The listing builds one solid part. Answer for the finished solid, in the listing's coordinates (mm). Face numbers are marked on the shaded views. A direction names the side the tool comes from. Give positions to 0.01 mm unless a question says otherwise; leave off trailing zeros. Write each loop counter-clockwise with the first axis right and the second up, starting at its lowest first coordinate (ties: lowest second). Pieces come first, ordered by that corner, then holes. Notation, with made-up numbers: M 52,71.5 L 75,71.5 A23 ccw 75,99.5 Z; hole C -15,33 d10. An arc over 180 degrees is marked long. Return JSON: item names as keys, results as strings.
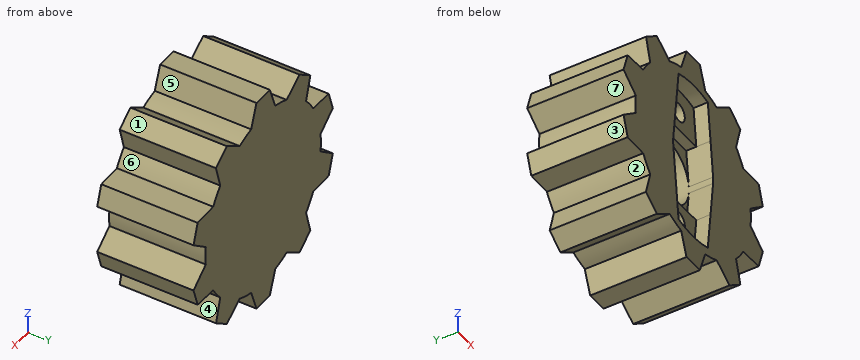
from build123d import *

# Parameters (mm, degrees)
CROQUIS1_R              = 3.75
SALIENTE_EXTRUIR1_DEPTH = 11.5
CROQUIS1_4_R            = 1.1
CORTAR_EXTRUIR1_DEPTH   = 1.7
CORTAR_EXTRUIR2_START   = 1.7
CORTAR_EXTRUIR2_DEPTH   = 1.2
CUT_EXTRUDE1_START      = 1.7
CROQUIS1_7_R            = 1.1
CUT_EXTRUDE1_DEPTH      = 6.5
BOSS_EXTRUDE1_START     = 11.5
BOSS_EXTRUDE1_DEPTH     = 5.6


with BuildPart() as part:
    # Croquis1 → Saliente-Extruir1 (new body)
    with BuildSketch(Plane(origin=(0, 0, 0), x_dir=(1, 0, 0), z_dir=(0, 1, 0))):
        with BuildLine():
            Line((1.248257156, 13.300370373), (-1.251742735, 13.299629349))
            Line((-1.251742735, 13.299629349), (-2.247599184, 10.563536241))
            ThreePointArc((-2.247599184, 10.563536241), (-3.339078028, 10.270859649), (-4.394000333, 9.865736722))
            Line((-4.394000333, 9.865736722), (-6.807900303, 11.493932811))
            Line((-6.807900303, 11.493932811), (-8.830007137, 10.023870243))
            Line((-8.830007137, 10.023870243), (-8.027436751, 7.224974686))
            ThreePointArc((-8.027436751, 7.224974686), (-8.7384307, 6.346639181), (-9.353755491, 5.398820076))
            Line((-9.353755491, 5.398820076), (-12.263671238, 5.297203579))
            Line((-12.263671238, 5.297203579), (-13.035508935, 2.919333403))
            Line((-13.035508935, 2.919333403), (-10.741066321, 1.126718369))
            ThreePointArc((-10.741066321, 1.126718369), (-10.799999853, -0.001781739), (-10.740693974, -1.13026234))
            Line((-10.740693974, -1.13026234), (-13.035136587, -2.922877375))
            Line((-13.035136587, -2.922877375), (-12.261889379, -5.300289572))
            Line((-12.261889379, -5.300289572), (-9.351973632, -5.401906069))
            ThreePointArc((-9.351973632, -5.401906069), (-8.73633614, -6.349522096), (-8.025052421, -7.227622959))
            Line((-8.025052421, -7.227622959), (-8.827622808, -10.026518516))
            Line((-8.827622808, -10.026518516), (-6.804644848, -11.495382082))
            Line((-6.804644848, -11.495382082), (-4.390744878, -9.867185993))
            ThreePointArc((-4.390744878, -9.867185993), (-3.335688959, -10.271960824), (-2.244113605, -10.564277265))
            Line((-2.244113605, -10.564277265), (-1.248257156, -13.300370373))
            Line((-1.248257156, -13.300370373), (1.251742735, -13.299629349))
            Line((1.251742735, -13.299629349), (2.247599184, -10.563536241))
            ThreePointArc((2.247599184, -10.563536241), (3.339078028, -10.270859649), (4.394000333, -9.865736722))
            Line((4.394000333, -9.865736722), (6.807900303, -11.493932811))
            Line((6.807900303, -11.493932811), (8.830007137, -10.023870243))
            Line((8.830007137, -10.023870243), (8.027436751, -7.224974686))
            ThreePointArc((8.027436751, -7.224974686), (8.7384307, -6.346639181), (9.353755491, -5.398820076))
            Line((9.353755491, -5.398820076), (12.263671238, -5.297203579))
            Line((12.263671238, -5.297203579), (13.035508935, -2.919333403))
            Line((13.035508935, -2.919333403), (10.741066321, -1.126718369))
            ThreePointArc((10.741066321, -1.126718369), (10.799999853, 0.001781739), (10.740693974, 1.13026234))
            Line((10.740693974, 1.13026234), (13.035136587, 2.922877375))
            Line((13.035136587, 2.922877375), (12.261889379, 5.300289572))
            Line((12.261889379, 5.300289572), (9.351973632, 5.401906069))
            ThreePointArc((9.351973632, 5.401906069), (8.73633614, 6.349522096), (8.025052421, 7.227622959))
            Line((8.025052421, 7.227622959), (8.827622808, 10.026518516))
            Line((8.827622808, 10.026518516), (6.804644848, 11.495382082))
            Line((6.804644848, 11.495382082), (4.390744878, 9.867185993))
            ThreePointArc((4.390744878, 9.867185993), (3.335688959, 10.271960824), (2.244113605, 10.564277265))
            Line((2.244113605, 10.564277265), (1.248257156, 13.300370373))
        make_face()
        with Locations(Location((0, 0, 0), (0, 0, 270))):
            Circle(CROQUIS1_R, mode=Mode.SUBTRACT)
    extrude(amount=SALIENTE_EXTRUIR1_DEPTH)

    # Croquis1<4> → Cortar-Extruir1 (cut)
    with BuildSketch(Plane(origin=(0, 0, 0), x_dir=(1, 0, 0), z_dir=(0, 1, 0))):
        with BuildLine():
            ThreePointArc((3.727502093, -0.41015625), (0, -3.75), (-3.727502093, -0.41015625))
            Line((-3.727502093, -0.41015625), (-3.249966737, -4.75))
            Line((-3.249966737, -4.75), (3.249966737, -4.75))
            Line((3.249966737, -4.75), (3.727502093, -0.41015625))
        make_face()
        with BuildLine():
            Line((3.249966737, -4.75), (-3.249966737, -4.75))
            Line((-3.249966737, -4.75), (-2.737205389, -9.409977746))
            ThreePointArc((-2.737205389, -9.409977746), (0, -9.7999987), (2.737205389, -9.409977746))
            Line((2.737205389, -9.409977746), (3.249966737, -4.75))
        make_face()
        with Locations((0, -7)):
            Circle(CROQUIS1_4_R, mode=Mode.SUBTRACT)
        with BuildLine():
            Line((3.248223947, 4.75), (-3.251709526, 4.75))
            Line((-3.251709526, 4.75), (-3.727664518, 0.408677426))
            ThreePointArc((-3.727664518, 0.408677426), (-0.001487905, 3.749999705), (3.727339039, 0.411635384))
            Line((3.727339039, 0.411635384), (3.248223947, 4.75))
        make_face()
        with BuildLine():
            Line((-2.740938342, 9.408891089), (-3.251709526, 4.75))
            Line((-3.251709526, 4.75), (3.248223947, 4.75))
            Line((3.248223947, 4.75), (2.733471058, 9.411063197))
            ThreePointArc((2.733471058, 9.411063197), (-0.003888392, 9.799997928), (-2.740938342, 9.408891089))
        make_face()
        with Locations((0, 7)):
            Circle(CROQUIS1_4_R, mode=Mode.SUBTRACT)
        with Locations((0, 7)):
            Circle(CROQUIS1_4_R)
        with Locations((0, -7)):
            Circle(CROQUIS1_4_R)
    extrude(amount=CORTAR_EXTRUIR1_DEPTH, mode=Mode.SUBTRACT)

    # Croquis1<5> → Cortar-Extruir2 (cut)
    with BuildSketch(Plane(origin=(0, 0, 0), x_dir=(1, 0, 0), z_dir=(0, 1, 0)).offset(CORTAR_EXTRUIR2_START)):
        with BuildLine():
            Line((3.248223947, 4.75), (-3.251709526, 4.75))
            Line((-3.251709526, 4.75), (-3.727664518, 0.408677426))
            ThreePointArc((-3.727664518, 0.408677426), (-0.001487905, 3.749999705), (3.727339039, 0.411635384))
            Line((3.727339039, 0.411635384), (3.248223947, 4.75))
        make_face()
        with BuildLine():
            ThreePointArc((3.727502093, -0.41015625), (0, -3.75), (-3.727502093, -0.41015625))
            Line((-3.727502093, -0.41015625), (-3.249966737, -4.75))
            Line((-3.249966737, -4.75), (3.249966737, -4.75))
            Line((3.249966737, -4.75), (3.727502093, -0.41015625))
        make_face()
    extrude(amount=CORTAR_EXTRUIR2_DEPTH, mode=Mode.SUBTRACT)

    # Croquis1<7> → Cut-Extrude1 (cut)
    with BuildSketch(Plane(origin=(0, 0, 0), x_dir=(1, 0, 0), z_dir=(0, 1, 0)).offset(CUT_EXTRUDE1_START)):
        with Locations(Location((0, -7, 0), (0, 0, 90))):
            Circle(CROQUIS1_7_R)
        with Locations(Location((0, 7, 0), (0, 0, 90))):
            Circle(CROQUIS1_7_R)
    extrude(amount=CUT_EXTRUDE1_DEPTH, mode=Mode.SUBTRACT)

    # Croquis1<10> → Boss-Extrude1 (add)
    with BuildSketch(Plane(origin=(0, 0, 0), x_dir=(1, 0, 0), z_dir=(0, 1, 0)).offset(BOSS_EXTRUDE1_START)):
        with BuildLine():
            ThreePointArc((0, 1.6), (-1.6, 0), (0, -1.6))
            Line((0, -1.6), (0, 1.6))
        make_face()
        with BuildLine():
            Line((0, 1.6), (0, -1.6))
            ThreePointArc((0, -1.6), (1.13137085, -1.13137085), (1.6, 0))
            ThreePointArc((1.6, 0), (1.13137085, 1.13137085), (0, 1.6))
        make_face()
        with BuildLine():
            ThreePointArc((0, 2.6), (-2.6, 0), (0, -2.6))
            Line((0, -2.6), (0, -1.6))
            ThreePointArc((0, -1.6), (-1.6, 0), (0, 1.6))
            Line((0, 1.6), (0, 2.6))
        make_face()
        with BuildLine():
            Line((0, -1.6), (0, -2.6))
            ThreePointArc((0, -2.6), (1.838477631, -1.838477631), (2.6, 0))
            ThreePointArc((2.6, 0), (1.838477631, 1.838477631), (0, 2.6))
            Line((0, 2.6), (0, 1.6))
            ThreePointArc((0, 1.6), (1.13137085, 1.13137085), (1.6, 0))
            ThreePointArc((1.6, 0), (1.13137085, -1.13137085), (0, -1.6))
        make_face()
        with BuildLine():
            ThreePointArc((-3.727502093, -0.41015625), (-2.502440215, -2.792900458), (0, -3.75))
            Line((0, -3.75), (0, -2.6))
            ThreePointArc((0, -2.6), (-2.6, 0), (0, 2.6))
            Line((0, 2.6), (0, 3.75))
            ThreePointArc((0, 3.75), (-2.502994172, 2.792404013), (-3.727664518, 0.408677426))
            ThreePointArc((-3.727664518, 0.408677426), (-3.749999926, -0.000743858), (-3.727502093, -0.41015625))
        make_face()
        with BuildLine():
            Line((0, -2.6), (0, -3.75))
            ThreePointArc((0, -3.75), (2.502440215, -2.792900458), (3.727502093, -0.41015625))
            ThreePointArc((3.727502093, -0.41015625), (3.744371299, -0.205386407), (3.75, 0))
            ThreePointArc((3.75, 0), (3.744330474, 0.206129334), (3.727339039, 0.411635384))
            ThreePointArc((3.727339039, 0.411635384), (2.50188602, 2.793396919), (0, 3.75))
            Line((0, 3.75), (0, 2.6))
            ThreePointArc((0, 2.6), (1.838477631, 1.838477631), (2.6, 0))
            ThreePointArc((2.6, 0), (1.838477631, -1.838477631), (0, -2.6))
        make_face()
    extrude(amount=-BOSS_EXTRUDE1_DEPTH)


solid = part.part
Item 1: A cutting plane is placed at B-B, the plane x = 0. Write down the section's boundary in (y, z), plus the area to 3 significant figures.
Geometry results:
{"outline": "M 0,-13.3 L 11.5,-13.3 L 11.5,13.3 L 0,13.3 L 0,9.8 L 1.7,9.8 L 1.7,8.1 L 8.2,8.1 L 8.2,5.9 L 1.7,5.9 L 1.7,4.75 L 2.9,4.75 L 2.9,3.75 L 5.9,3.75 L 5.9,-3.75 L 2.9,-3.75 L 2.9,-4.75 L 1.7,-4.75 L 1.7,-5.9 L 8.2,-5.9 L 8.2,-8.1 L 1.7,-8.1 L 1.7,-9.8 L 0,-9.8 Z", "area": "210 mm2"}
Item 2: A cutting plane is placed at C-C, the plane z = 0. Write down the section's boundary in (x, y), plus the area to 3 significant figures.
Geometry results:
{"outline": "M -10.8,0 L -3.75,0 L -3.75,5.9 L 3.75,5.9 L 3.75,0 L 10.8,0 L 10.8,11.5 L -10.8,11.5 Z", "area": "204 mm2"}
Item 3: Determine the mould class of the marked faces 1, 2, 3 and 4 for opening direction Z: +Z half, -Z half, draft (parallel to the pull), parting line (faces both ways), or undercut.
Geometry results:
{"face 1": "+Z half", "face 2": "undercut", "face 3": "-Z half", "face 4": "undercut"}
Item 4: Given pin 1 Ø5.5 at (x, z) = (0.5, -8.5) entering from -Y; pin 2 Ø0.7 at (x, z) = (-0.5, -6.5) entering from -Y; pin 3 Ø3.5 at (x, z) = (1.5, -2) entering from -Y; pin 4 Ø1 at (y, z) = (7.5, 2) entering from -X, each flat-ended and moving along its own axis, determine where each tip first touches the part or whether it passes through.
Geometry results:
{"pin 1": "stops at y = 0", "pin 2": "stops at y = 8.2", "pin 3": "stops at y = 2.9", "pin 4": "stops at x = -12.49"}
Item 5: A cutting plane is placed at A-A, the plane x = 11.25. Write down the section's boundary in (y, z).
Geometry results:
{"outline": "M 0,-5.34 L 11.5,-5.34 L 11.5,-1.53 L 0,-1.53 Z; M 0,1.52 L 11.5,1.52 L 11.5,5.33 L 0,5.33 Z"}
Item 6: A cutting plane is placed at D-D, the plane y = 6.5. Count the separate pieces of the cut face and the enclosed holes in it, plus the area to 3 significant figures.
Geometry results:
{"separate pieces": "1", "enclosed holes": "2", "area": "447 mm2"}
Item 7: Find the intervals of material crossed by line 1 (X direction, y = 4.6, z = 0); line 2 (X direction, y = 2.5, z = -11); line 3 (Y direction, x = -2.5, z = -7.5), in increasing order.
Geometry results:
{"line 1": "x = -10.8 to -3.75, 3.75 to 10.8", "line 2": "x = -7.49 to -6.08, -2.09 to 2.09, 6.07 to 7.49", "line 3": "y = 1.7 to 11.5"}
Item 8: Which of the six approach directions +Z, -Z, +X, -X, +Y, -Y give full straight-line access (tool end or side, diameter ignored) to the marked faces 5, 6 and 7?
Geometry results:
{"face 5": "+Z, +Y, -Y", "face 6": "+X, +Y, -Y", "face 7": "-X, +Y, -Y"}
